Part model, mm, in its own coordinate system. Face numbers are marked on the shaded views. A direction names the side the tool comes from. Give positions to 0.01 mm unless a question says otherwise; leave off trailing zeros. Order: outer loops, then holes, each group sorted by start corner. A loop starts at its lowest first (then second) coordinate and runs counter-clockwise, first axis right, second up.
1. Slice it at C-C on x = -6.5. List the corners of the cut face in (y, z), and give its area (3 significant figures).
2. Slice it at A-A on y = 80. List the corners of the cut face in (x, z), and give its area (3 significant figures).
3. Probe line 1 (Z direction, x = 181, y = 26); line 2 (X direction, y = 49, z = 44); line 3 (Y direction, x = 61, z = -20.5). List the from-to ranges inside material, lowest first.
4. Slice it at B-B on z = 9. List the corners of the cut face in (x, y).
5. Which spindle directions (+Z, -Z, +X, -X, +Y, -Y) get a long thin tool onto all of the face, cutting with end or side? Do the marked faces 1 and 2. Say none if no direction does.
6. Drop a flat-ended pin along its axis: pin 1 Ø12 at (x, z) = (134.5, 25.5) entering from -Y. Give the stop position or say it passes through.
7. Mould opens along Z. For the marked faces 3, 4 and 5 say: +Z half, -Z half, draft (parallel to the pull), parting line (faces both ways), or undercut.
from build123d import *

# Parameters (mm, degrees)
BOSS_EXTRUDE1_DEPTH = 100
SHELL1_T            = -5


with BuildPart() as part:
    # Sketch1 → Boss-Extrude1 (new body)
    with BuildSketch(Plane(origin=(0, 0, 0), x_dir=(1, 0, 0), z_dir=(0, 1, 0))):
        with BuildLine():
            Line((-235, -75), (235, -75))
            ThreePointArc((235, -75), (245.606601718, -70.606601718), (250, -60))
            Line((250, -60), (250, 60))
            ThreePointArc((250, 60), (245.606601718, 70.606601718), (235, 75))
            Line((235, 75), (-235, 75))
            ThreePointArc((-235, 75), (-245.606601718, 70.606601718), (-250, 60))
            Line((-250, 60), (-250, -60))
            ThreePointArc((-250, -60), (-245.606601718, -70.606601718), (-235, -75))
        make_face()
    extrude(amount=BOSS_EXTRUDE1_DEPTH)

    # Shell1
    shell1_openings = [part.faces().sort_by_distance(p)[0] for p in [
        (0, 0, 0),
    ]]
    offset(amount=SHELL1_T, openings=shell1_openings, kind=Kind.INTERSECTION)


solid = part.part
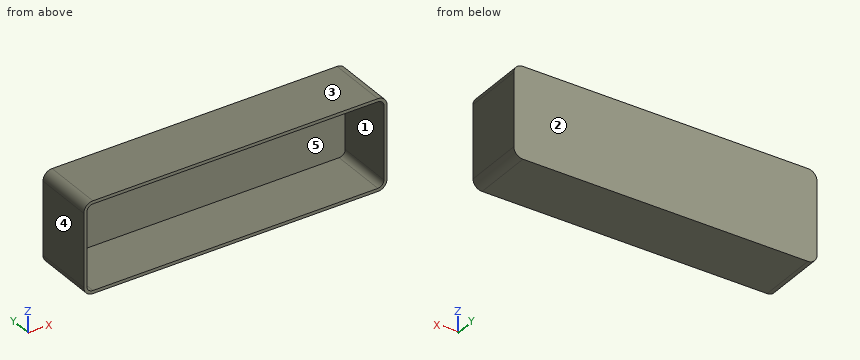
Data:
1. outline: (0, -75) - (100, -75) - (100, 75) - (0, 75) - (0, 70) - (95, 70) - (95, -70) - (0, -70) - close
1. area: 1,700 mm2
2. outline: (-250, -60) arc R15 ccw to (-235, -75) - (235, -75) arc R15 ccw to (250, -60) - (250, 60) arc R15 ccw to (235, 75) - (-235, 75) arc R15 ccw to (-250, 60) - close; hole (-245, -60) arc R10 ccw to (-235, -70) - (235, -70) arc R10 ccw to (245, -60) - (245, 60) arc R10 ccw to (235, 70) - (-235, 70) arc R10 ccw to (-245, 60) - close
2. area: 6,290 mm2
3. line 1: z = -75 to -70, 70 to 75
3. line 2: x = -250 to -245, 245 to 250
3. line 3: y = 95 to 100
4. outline: (-250, 0) - (-245, 0) - (-245, 95) - (245, 95) - (245, 0) - (250, 0) - (250, 100) - (-250, 100) - close
5. face 1: -Y
5. face 2: +Z, -Z, +X, -X, +Y
6. pin 1: stops at y = 95
7. face 3: +Z half
7. face 4: draft
7. face 5: undercut
